Could you check a few things on this model? Use its own coordinates, in mm. A direction names the side the tool comes from. Give positions to 0.01 mm unless a question says otherwise; leave off trailing zeros. Write each loop counter-clockwise with the first axis right and the second up, starting at its lowest first coordinate (ties: lowest second). Pieces come first, ordered by that corner, then holes. Notation, with made-up numbers: M 26,65 L 36,65 A25 cw 36,87 Z; hole C 45,-39 d1. An arc over 180 degrees is marked long. One line per item, written item: value.
```python
from build123d import *

# Parameters (mm, degrees)
SKETCH1_R           = 11.5
BOSS_EXTRUDE1_DEPTH = 19
SKETCH2_R           = 1
SKETCH2_R_2         = 3.25
CUT_EXTRUDE1_DEPTH  = 8.5


with BuildPart() as part:
    # Sketch1 → Boss-Extrude1 (new body)
    with BuildSketch(Plane(origin=(0, 0, 0), x_dir=(1, 0, 0), z_dir=(0, 1, 0))):
        Circle(SKETCH1_R)
    extrude(amount=BOSS_EXTRUDE1_DEPTH)

    # Sketch2 → Cut-Extrude1 (cut)
    with BuildSketch(Plane(origin=(0, 19, 0), x_dir=(1, 0, 0), z_dir=(0, 1, 0))):
        with Locations((0, 8.5)):
            Circle(SKETCH2_R)
        with Locations((0, -8.5)):
            Circle(SKETCH2_R)
        Circle(SKETCH2_R_2)
    extrude(amount=-CUT_EXTRUDE1_DEPTH, mode=Mode.SUBTRACT)


solid = part.part
```
1) If we section it at B-B, the plane x = 0: Write out the boundary of the cut face in (y, z).
Outcome:
outline: M 0,-11.5 L 19,-11.5 L 19,-9.5 L 10.5,-9.5 L 10.5,-7.5 L 19,-7.5 L 19,-3.25 L 10.5,-3.25 L 10.5,3.25 L 19,3.25 L 19,7.5 L 10.5,7.5 L 10.5,9.5 L 19,9.5 L 19,11.5 L 0,11.5 Z
2) I'm going to push flat-ended pins straight in: pin 1 (1 mm diameter, centred on x = -2, y = 11, fed in from +Z); pin 2 (5 mm diameter, centred on x = 5, y = 9.5, fed in from +Z) (3 decimals); pin 3 (8 mm diameter, centred on x = -8.5, y = 10.5, fed in from +Z). Where does each tip first touch, or does it pass through?
Outcome:
pin 1: stops at z = 11.4
pin 2: stops at z = 11.225
pin 3: stops at z = 10.58
3) If we section it at D-D, the plane y = 9.5: Write out the boundary of the cut face in (x, z).
Outcome:
outline: C 0,0 d23
4) We'd pull the mould along Z, two halves only. Please class faces 1 (the face through (-1.5, 9.4, -11.4)), 2 (the face through (-3, 19, 2)), 3 (the face through (-2.579, 14.81, 1.978)): pulls with the +Z half, pulls with the -Z half, needs draft (parallel to the pull), parting line crosses it, or undercut.
Outcome:
face 1: parting line crosses it
face 2: needs draft
face 3: undercut
5) If we section it at C-C, the plane y = 13.75: Write out the boundary of the cut face in (x, z).
Outcome:
outline: C 0,0 d23; hole C 0,0 d6.5; hole C 0,-8.5 d2; hole C 0,8.5 d2
6) If we section it at A-A, the plane z = 0: Write out the boundary of the cut face in (x, y), then the cut area to 3 significant figures.
Outcome:
outline: M -11.5,0 L 11.5,0 L 11.5,19 L 3.25,19 L 3.25,10.5 L -3.25,10.5 L -3.25,19 L -11.5,19 Z
area: 382 mm^2
7) On a 3-axis mill with a long thin cutter (end or side, diameter ignored), from which of +Z, -Z, +X, -X, +Y, -Y can I reach the whole of each face in a straight line? I mean faces 4 (the face through (0, 0, 0)), 5 (the face through (0, 10.5, -9)). Say none if no direction works.
Outcome:
face 4: +Z, -Z, +X, -X, -Y
face 5: +Y
8) Please list where these lines run through material, in increasing order: L1, parallel to Z at x = 0, y = 15.75; L2, parallel to X at y = 12.75, z = 0; L3, parallel to X at y = 13.75, z = 8.5. Write a range as from..to.
Outcome:
L1: z = -11.5..-9.5, -7.5..-3.25, 3.25..7.5, 9.5..11.5
L2: x = -11.5..-3.25, 3.25..11.5
L3: x = -7.75..-1, 1..7.75
